from build123d import *

# Parameters (mm, degrees)
CROQUIS1_R              = 12
CROQUIS1_R_2            = 1.6
CROQUIS1_R_3            = 3.5
SALIENTE_EXTRUIR1_DEPTH = 3
CROQUIS2_R              = 6
CROQUIS2_R_2            = 3
SALIENTE_EXTRUIR2_DEPTH = 12.95
CROQUIS3_R              = 4.05
CROQUIS3_R_2            = 3
SALIENTE_EXTRUIR3_DEPTH = 9
REDONDEO1_R             = 0.5


with BuildPart() as part:
    # Croquis1 → Saliente-Extruir1 (new body)
    with BuildSketch(Plane(origin=(0, 0, 0), x_dir=(0, 1, 0), z_dir=(0, 0, 1))):
        with Locations(Location((0, 0, 0), (0, 0, 270))):
            Circle(CROQUIS1_R)
        with Locations(Location((0, 9, 0), (0, 0, 270))):
            Circle(CROQUIS1_R_2, mode=Mode.SUBTRACT)
        with Locations(Location((7.794228634, -4.5, 0), (0, 0, 270))):
            Circle(CROQUIS1_R_2, mode=Mode.SUBTRACT)
        with Locations(Location((-7.794228634, -4.5, 0), (0, 0, 270))):
            Circle(CROQUIS1_R_2, mode=Mode.SUBTRACT)
        with Locations(Location((0, 0, 0), (0, 0, 270))):
            Circle(CROQUIS1_R_3, mode=Mode.SUBTRACT)
    extrude(amount=SALIENTE_EXTRUIR1_DEPTH)

    # Croquis2 → Saliente-Extruir2 (add)
    with BuildSketch(Plane.XY.offset(3)):
        with Locations(Location((0, 0, 0), (0, 0, 180))):
            Circle(CROQUIS2_R)
        with Locations(Location((0, 0, 0), (0, 0, 180))):
            Circle(CROQUIS2_R_2, mode=Mode.SUBTRACT)
    extrude(amount=SALIENTE_EXTRUIR2_DEPTH)

    # Croquis3 → Saliente-Extruir3 (add)
    with BuildSketch(Plane.XY.offset(15.95)):
        Circle(CROQUIS3_R)
        with Locations(Location((0, 0, 0), (0, 0, 180))):
            Circle(CROQUIS3_R_2, mode=Mode.SUBTRACT)
    extrude(amount=SALIENTE_EXTRUIR3_DEPTH)

    # Redondeo1
    redondeo1_edges = [part.edges().sort_by_distance(p)[0] for p in [
        (6, 0, 3),
        (6, 0, 15.95),
        (-4.05, 0, 24.95),
        (3, 0, 24.95),
    ]]
    fillet(redondeo1_edges, radius=REDONDEO1_R)


solid = part.part
For this review, take the finished solid that the model builds, in its own axes (mm). A direction names the side the tool comes from. Coordinates: 2 decimals unless noted, no trailing zeros. Loops run counter-clockwise (first coordinate to the right, second up) from the corner with the lowest first, then second, coordinate; pieces in that order, holes last. Notation, with made-up numbers: (83, 2) -> (136, 2) arc R13 ccw to (136, 24) -> close; hole circle Ø3 at (29, 58). An arc over 180 degrees is marked (long way). Write each question's results on one line, items separated by ' | '.
Q1. Add section D-D, the plane z = 10.25. State the section outline as (x, y) points, then the cut area to 3 significant figures.
Taken from the geometry:
outline: circle Ø12 at (0, 0); hole circle Ø6 at (0, 0) | area: 84.8 mm²
Q2. Add section A-A, the plane y = 0. Count the separate pieces of the cut face and the enclosed holes in it, then the cut area to 3 significant figures.
Taken from the geometry:
separate pieces: 3 | enclosed holes: 0 | area: 138 mm²
Q3. Mouldability with a two-part tool opening along Y and no side actions: class faces 4 (the cylindrical face through (-5.723, -1.802, 9.391)), 5 (the cylindrical face through (6.026, 8.275, 1.479)), 6 (the flat face through (-2.8, -2.5, 0)) as +Y half, -Y half, draft (parallel to the pull), parting line (faces both ways), or undercut.
Taken from the geometry:
face 4: parting line | face 5: undercut | face 6: draft
Q4. Machinability: for faces 1 (the cylindrical face through (-10.6, 0.07, 1.48)), 2 (the flat face through (-3, -1, 3)), 3 (the flat face through (5, -5, 3)), which of the approach directions +Z, -Z, +X, -X, +Y, -Y give a long, thin tool a straight path to every point of the face, cutting with its end or side? Answer none if there is none.
Taken from the geometry:
face 1: +Z, -Z | face 2: -Z | face 3: +Z
Q5. To check wall thickness, follow line 1 along Y through (x, z) = (0, 1.2); line 2 along Y through (x, z) = (4.5, 1.5); line 3 along Z through (x, y) = (0, -5). State the ranges of each line that lie inside material, in increasing order. Write a range as [from, to].
Taken from the geometry:
line 1: [-12, -3.5], [3.5, 12] | line 2: [-11.12, -9.39], [-6.19, 6.19], [9.39, 11.12] | line 3: [0, 15.95]
Q6. Add section B-B, the plane x = 0. State the section outline as (y, z) points, then the cut area to 3 significant figures.
Taken from the geometry:
outline: (-12, 0) -> (-3.5, 0) -> (-3.5, 3) -> (-3, 3) -> (-3, 24.45) arc R0.5 ccw to (-3.5, 24.95) -> (-3.55, 24.95) arc R0.5 ccw to (-4.05, 24.45) -> (-4.05, 15.95) -> (-5.5, 15.95) arc R0.5 ccw to (-6, 15.45) -> (-6, 3.5) arc R0.5 cw to (-6.5, 3) -> (-12, 3) -> close; (3, 3) -> (3.5, 3) -> (3.5, 0) -> (12, 0) -> (12, 3) -> (6.5, 3) arc R0.5 cw to (6, 3.5) -> (6, 15.45) arc R0.5 ccw to (5.5, 15.95) -> (4.05, 15.95) -> (4.05, 24.45) arc R0.5 ccw to (3.55, 24.95) -> (3.5, 24.95) arc R0.5 ccw to (3, 24.45) -> close | area: 147 mm²
Q7. For pin 1 Ø1 at (x, y) = (0.5, 8) entering from +Z; pin 2 Ø12 at (x, y) = (4.5, 1.5) entering from +Z; pin 3 Ø2.5 at (x, y) = (-9, 0) entering from +Z; pin 4 Ø1 at (x, z) = (4, 21.5) entering from -Y, all flat-tipped, find the tip position at first contact; note any pin that passes through.
Taken from the geometry:
pin 1: z = 3 | pin 2: z = 24.95 | pin 3: through | pin 4: y = -2.04
Q8. Add section C-C, the plane y = 8.25. State the section outline as (x, z) points.
Taken from the geometry:
outline: (-8.71, 0) -> (2.97, 0) -> (2.97, 3) -> (-8.71, 3) -> close; (6.03, 0) -> (8.71, 0) -> (8.71, 3) -> (6.03, 3) -> close
